Input: part model. Units: mm. Frame: model coordinates. A direction names the side the tool comes from. Give positions to 0.01 mm unless a question says otherwise; leave off trailing zeros. Loops run counter-clockwise (first coordinate to the right, second up) from the corner with the lowest first, then second, coordinate; pieces in that order, holes last. Notation, with made-up numbers: M 66,-29 L 99,-29 A27 ccw 99,9 Z; hole C -40,-18.5 d4. An arc over 180 degrees is marked long. Use CSV: the item, a comma, the result in double quotes. Start each with the question number.
Q1. Pull-direction query (Z, two-part tool) for faces 1 (the cylindrical face through (-473.89, 196.02, -175.78)), 2 (the cylindrical face through (170.22, 25.35, -169.25)), 3 (the cylindrical face through (-473.89, 68.72, 2.72)); classes: released by +Z, released by -Z, zero draft, split by the parting line, or undercut.
Q2. Section C-C, the plane z = -163.5. Output: boundary loops of the cut face in (x, y).
Q3. Material intervals for line 1 along Y through (x, z) = (-303, 9.5); line 2 along Y through (x, z) = (468, 84.5); line 3 along X through (y, z) = (181.5, -152), sorted ascending.
Q4. Pin query (flat end, axial travel): pin 1 (10 mm diameter, centred on x = 368.5, z = -140.5, fed in from -Y); pin 2 (3 mm diameter, centred on y = 107, z = 148.5, fed in from -X); pin 3 (12 mm diameter, centred on y = 266, z = -93.5, fed in from +X). Return the tip coordinate at first contact, or that it passes through.
Q5. Section B-B, the plane x = -361.5. Output: boundary loops of the cut face in (y, z), plus the area to 3 significant figures.
Q6. Section D-D, the plane x = 422. Output: boundary loops of the cut face in (y, z).
Q7. Reachability of faces 4 (the cylindrical face through (-329.62, 25.35, -162.84)), 5 (the flat face through (-40, 338, 3)) from +Z, -Z, +X, -X, +Y, -Y: full face, straight path, thin tool, end or side. Return the list, or none.
Q8. Section A-A, the plane z = -32. Output: boundary loops of the cut face in (x, y).
from build123d import *

# Parameters (mm, degrees)
F1_W     = 1044
F1_H     = 389
F2_DEPTH = 288
F3_R     = 100
F5_DEPTH = 389.001
F6_R     = 15
F7_DEPTH = 50


with BuildPart() as f2:
    # F1 (on Front) → F2 (new body)
    with BuildSketch(Plane.XZ):
        with Locations((6.3670966774, 0)):
            Rectangle(F1_W, F1_H)
    extrude(amount=-F2_DEPTH)

    # F3
    f3_edges = [f2.edges().sort_by_distance(p)[0] for p in [
        (-515.632903, 144, 194.5),
        (-515.632903, 144, -194.5),
        (-515.632903, 0, 0),
        (-515.632903, 288, 0),
    ]]
    fillet(f3_edges, radius=F3_R)

    # F4 (on face) → F5 (cut, through all)
    with BuildSketch(Plane.XY.offset(194.5)):
        Polygon((528.3670966774, 288), (346.5153428453, 288), (528.3670966774, 160.6660311301), align=None)
    extrude(amount=-F5_DEPTH, mode=Mode.SUBTRACT)

    # F6 (on face) → F7 (join)
    with BuildSketch(Plane.XZ):
        with Locations((-314.6329033226, 163.5)):
            Circle(F6_R)
        with Locations((156.3670966774, 163.5)):
            Circle(F6_R)
        with Locations((156.3670966774, -163.5)):
            Circle(F6_R)
        with Locations((-314.6329033226, -163.5)):
            Circle(F6_R)
    extrude(amount=F7_DEPTH)


with BuildPart() as f2_1:
    # F8: moved
    add(f2.part.moved(Location((0, 50, 0))))


solid = f2_1.part
A:
1,face 1,"released by -Z"
1,face 2,"undercut"
1,face 3,"zero draft"
2,outline,"M -488.01,81 A100 ccw -415.63,50 L -329.63,50 L -329.63,0 L -299.63,0 L -299.63,50 L 141.37,50 L 141.37,0 L 171.37,0 L 171.37,50 L 528.37,50 L 528.37,210.67 L 346.52,338 L -415.63,338 A100 ccw -488.01,307 Z"
3,line 1,"50 to 338"
3,line 2,"50 to 252.94"
3,line 3,"-497.45 to 528.37"
4,pin 1,"y = 50"
4,pin 2,"x = -500.74"
4,pin 3,"x = 457.91"
5,outline,"M 50,-194.5 L 338,-194.5 L 338,194.5 L 50,194.5 Z"
5,area,"112,000 mm^2"
6,outline,"M 50,-194.5 L 285.15,-194.5 L 285.15,194.5 L 50,194.5 Z"
7,face 4,"-Y"
7,face 5,"+Z, -Z, +X, -X, +Y"
8,outline,"M -515.63,150 A100 ccw -415.63,50 L 528.37,50 L 528.37,210.67 L 346.52,338 L -415.63,338 A100 ccw -515.63,238 Z"
